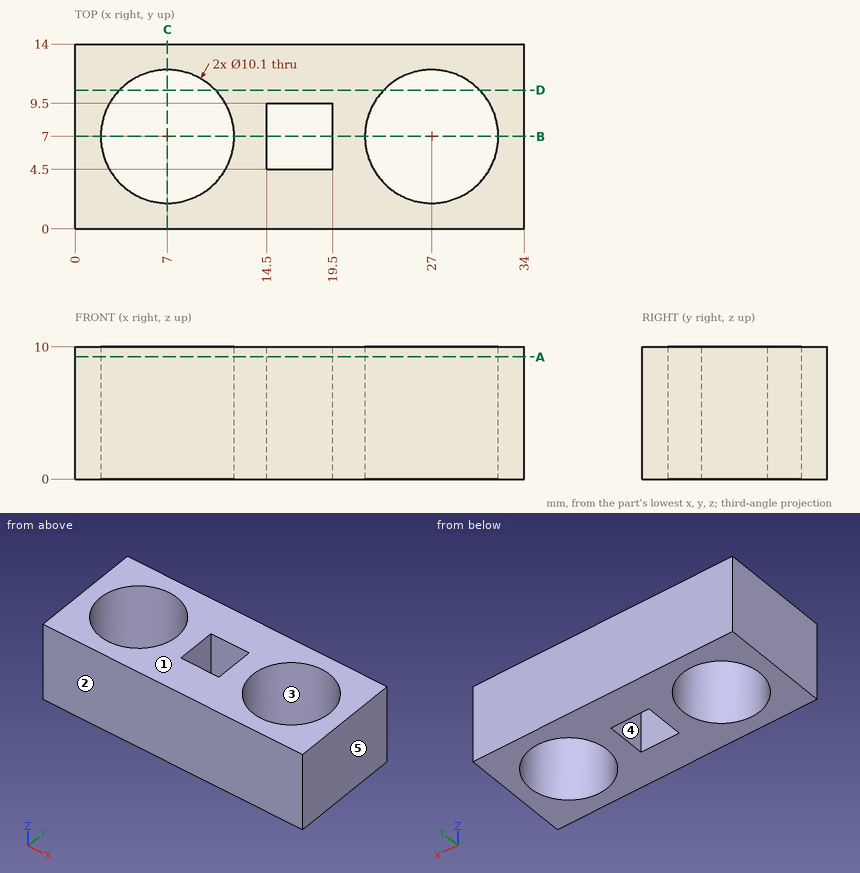
The drawing under review shows one solid part. Ordinate dimensions are in mm from its lowest x, y, z. A direction names the side the tool comes from. Round coordinates to 2 decimals unless told otherwise and drop trailing zeros. Loops run counter-clockwise (first coordinate to the right, second up) from the corner with the lowest first, then second, coordinate; pieces in that order, holes last. Notation, with made-up numbers: (73, -9) -> (79, -9) arc R15 cw to (79, 13) -> close; hole circle Ø9 at (88.25, 76.5). An arc over 180 degrees is marked (long way). One line per question, with ' | ' between items. Start each with the question number.
Item 1: Add section C-C, the plane x = 7. Write out the cut boundary in (y, z).
Item 2: Add section A-A, the plane z = 9.25. Write out the cut boundary in (x, y), then the cut area to 3 significant figures.
Item 3: Wall thickness on line 1 along Y through (x, z) = (19, 6.75); line 2 along X through (y, z) = (2.5, 4.75); line 3 along Y through (x, z) = (27, 7): over which ranges is each line inside the solid? List them lowest first. Write a range as [from, to].
Item 4: Add section B-B, the plane y = 7. Write out the cut boundary in (x, z).
Item 5: Machinability: for the marked faces 4 and 5, which of the approach directions +Z, -Z, +X, -X, +Y, -Y give a long, thin tool a straight path to every point of the face, cutting with its end or side? Answer none if there is none.
Item 6: Add section D-D, the plane y = 10.5. Write out the cut boundary in (x, z), then the cut area to 3 significant figures.
Item 7: Draft analysis for pull direction Y (two halves, no side actions). For the marked faces 1, 2 and 3, state which applies: +Y half, -Y half, draft (parallel to the pull), parting line (faces both ways), or undercut.
Return value:
1) outline: (0, 0) -> (1.95, 0) -> (1.95, 10) -> (0, 10) -> close; (12.05, 0) -> (14, 0) -> (14, 10) -> (12.05, 10) -> close
2) outline: (0, 0) -> (34, 0) -> (34, 14) -> (0, 14) -> close; hole circle Ø10.1 at (7, 7); hole (14.5, 4.5) -> (19.5, 4.5) -> (19.5, 9.5) -> (14.5, 9.5) -> close; hole circle Ø10.1 at (27, 7) | area: 291 mm2
3) line 1: y = [0, 4.5], [9.5, 14] | line 2: x = [0, 4.71], [9.29, 24.71], [29.29, 34] | line 3: y = [0, 1.95], [12.05, 14]
4) outline: (0, 0) -> (1.95, 0) -> (1.95, 10) -> (0, 10) -> close; (12.05, 0) -> (14.5, 0) -> (14.5, 10) -> (12.05, 10) -> close; (19.5, 0) -> (21.95, 0) -> (21.95, 10) -> (19.5, 10) -> close; (32.05, 0) -> (34, 0) -> (34, 10) -> (32.05, 10) -> close
5) face 4: +Z, -Z | face 5: +Z, -Z, +X, +Y, -Y
6) outline: (0, 0) -> (3.36, 0) -> (3.36, 10) -> (0, 10) -> close; (10.64, 0) -> (23.36, 0) -> (23.36, 10) -> (10.64, 10) -> close; (30.64, 0) -> (34, 0) -> (34, 10) -> (30.64, 10) -> close | area: 194 mm2
7) face 1: draft | face 2: -Y half | face 3: undercut
